For this review, take the finished solid that the model builds, in its own axes (mm). A direction names the side the tool comes from. Round coordinates to 2 decimals unless told otherwise and drop trailing zeros. Loops run counter-clockwise (first coordinate to the right, second up) from the corner with the lowest first, then second, coordinate; pieces in that order, holes last.
1. Tool access review of faces 1 (the cylindrical face through (0.488, -0.493, -0.108)), 2 (the cylindrical face through (-0.49, 29.49, -0.63)): name each direction out of +Z, -Z, +X, -X, +Y, -Y from which nothing blocks a thin tool from reaching the whole face with its end or side.
2. Consider section C-C on y = 4.5. State the section outline as (x, z) points, then the cut area to 3 significant figures.
3. Consider section B-B on x = 0. State the section outline as (y, z) points.
4. Consider section A-A on z = 0. State the section outline as (x, y) points, then the cut area to 3 significant figures.
5. Draft analysis for pull direction Y (two halves, no side actions). For faces 3 (the flat face through (0, 30, 0)), 4 (the cylindrical face through (-0.488, 28.507, -0.108)), 5 (the flat face through (0, -2, 0)), 6 (the cylindrical face through (-0.49, 13.8, -0.63)), state which applies: released by +Y, released by -Y, zero draft, split by the parting line, or undercut.
6. To check wall thickness, follow line 1 along Y through (x, z) = (-0.45, 0.4); line 2 along Z through (x, y) = (0.1, 10); line 3 along X through (y, z) = (21, -0.05). State the ranges of each line that lie inside material, in increasing order.
from build123d import *

# Parameters (mm, degrees)
SKETCH1_R           = 0.8
BOSS_EXTRUDE1_DEPTH = 30
SKETCH3_R           = 0.5
BOSS_EXTRUDE2_DEPTH = 1
SKETCH4_R           = 0.8
SKETCH4_R_2         = 0.5
CUT_EXTRUDE1_DEPTH  = 1
BOSS_EXTRUDE3_START = 1
SKETCH5_R           = 0.8
BOSS_EXTRUDE3_DEPTH = 1


with BuildPart() as part:
    # Sketch1 → Boss-Extrude1 (new body)
    with BuildSketch(Plane(origin=(0, 0, 0), x_dir=(1, 0, 0), z_dir=(0, 1, 0))):
        with Locations(Location((0, 0, 0), (0, 0, 270))):
            Circle(SKETCH1_R)
    extrude(amount=BOSS_EXTRUDE1_DEPTH)

    # Sketch3 → Boss-Extrude2 (add)
    with BuildSketch(Plane.XZ):
        with Locations(Location((0, 0, 0), (0, 0, 90))):
            Circle(SKETCH3_R)
    extrude(amount=BOSS_EXTRUDE2_DEPTH)

    # Sketch4 → Cut-Extrude1 (cut)
    with BuildSketch(Plane(origin=(0, 29, 0), x_dir=(1, 0, 0), z_dir=(0, 1, 0))):
        with Locations(Location((0, 0, 0), (0, 0, 270))):
            Circle(SKETCH4_R)
        with Locations(Location((0, 0, 0), (0, 0, 270))):
            Circle(SKETCH4_R_2, mode=Mode.SUBTRACT)
    extrude(amount=-CUT_EXTRUDE1_DEPTH, mode=Mode.SUBTRACT)

    # Sketch5 → Boss-Extrude3 (add)
    with BuildSketch(Plane.XZ.offset(1).offset(BOSS_EXTRUDE3_START)):
        with Locations(Location((0, 0, 0), (0, 0, 90))):
            Circle(SKETCH5_R)
    extrude(amount=-BOSS_EXTRUDE3_DEPTH)


solid = part.part
Resolved:
1. face 1: none
1. face 2: +Y, -Y
2. outline: circle Ø1.6 at (0, 0)
2. area: 2.01 mm2
3. outline: (-2, -0.8) - (-1, -0.8) - (-1, -0.5) - (0, -0.5) - (0, -0.8) - (28, -0.8) - (28, -0.5) - (29, -0.5) - (29, -0.8) - (30, -0.8) - (30, 0.8) - (29, 0.8) - (29, 0.5) - (28, 0.5) - (28, 0.8) - (0, 0.8) - (0, 0.5) - (-1, 0.5) - (-1, 0.8) - (-2, 0.8) - close
4. outline: (-0.8, -2) - (0.8, -2) - (0.8, -1) - (0.5, -1) - (0.5, 0) - (0.8, 0) - (0.8, 28) - (0.5, 28) - (0.5, 29) - (0.8, 29) - (0.8, 30) - (-0.8, 30) - (-0.8, 29) - (-0.5, 29) - (-0.5, 28) - (-0.8, 28) - (-0.8, 0) - (-0.5, 0) - (-0.5, -1) - (-0.8, -1) - close
4. area: 50.0 mm2
5. face 3: released by +Y
5. face 4: undercut
5. face 5: released by -Y
5. face 6: zero draft
6. line 1: y = -2 to -1, 0 to 28, 29 to 30
6. line 2: z = -0.79 to 0.79
6. line 3: x = -0.8 to 0.8
